Geometry check sheet. Reference: the model listing, model coordinates, mm. Give positions to 0.01 mm unless a question says otherwise; leave off trailing zeros. Write each loop counter-clockwise with the first axis right and the second up, starting at its lowest first coordinate (ties: lowest second). Pieces come first, ordered by that corner, then holes. Notation, with made-up numbers: (4, 46) -> (57, 46) arc R13 cw to (57, 55) -> close; hole circle Ø4 at (58, 70). An arc over 180 degrees is marked (long way). One line per item, written item: value.
from build123d import *

# Parameters (mm, degrees)
ESQUISSE1_W             = 10
ESQUISSE1_H             = 10
BOSS_EXTRU_1_DEPTH      = 95
ESQUISSE2_W             = 10
ESQUISSE2_H             = 5
BOSS_EXTRU_2_DEPTH      = 0.01
ESQUISSE3_W             = 10
ESQUISSE3_H             = 5
BOSS_EXTRU_3_DEPTH      = 0.01
ENL_V_MAT_EXTRU_2_DEPTH = 96.656155578


with BuildPart() as part:
    # Esquisse1 → Boss.-Extru.1 (new body)
    with BuildSketch(Plane.XY):
        Rectangle(ESQUISSE1_W, ESQUISSE1_H)
    extrude(amount=BOSS_EXTRU_1_DEPTH)

    # Esquisse2 → Boss.-Extru.2 (add)
    with BuildSketch(Plane(origin=(0, 5, 0), x_dir=(1, 0, 0), z_dir=(0, 1, 0))):
        with Locations((0, -92.5)):
            Rectangle(ESQUISSE2_W, ESQUISSE2_H)
    extrude(amount=BOSS_EXTRU_2_DEPTH)

    # Esquisse3 → Boss.-Extru.3 (add)
    with BuildSketch(Plane.XZ.offset(5)):
        with Locations((0, 2.5)):
            Rectangle(ESQUISSE3_W, ESQUISSE3_H)
    extrude(amount=BOSS_EXTRU_3_DEPTH)

    # Esquisse6 → Enlèv. mat.-Extru.2 (cut, through all)
    with BuildSketch(Plane(origin=(5, 0, 0), x_dir=(0, 0, -1), z_dir=(1, 0, 0))):
        with BuildLine():
            ThreePointArc((-27.625, 1.931491673), (-35.125, -0.005), (-27.625, -1.941491673))
            ThreePointArc((-27.625, -1.941491673), (-20.125, -0.005), (-27.625, 1.931491673))
        make_face()
    extrude(amount=-ENL_V_MAT_EXTRU_2_DEPTH, mode=Mode.SUBTRACT)


solid = part.part
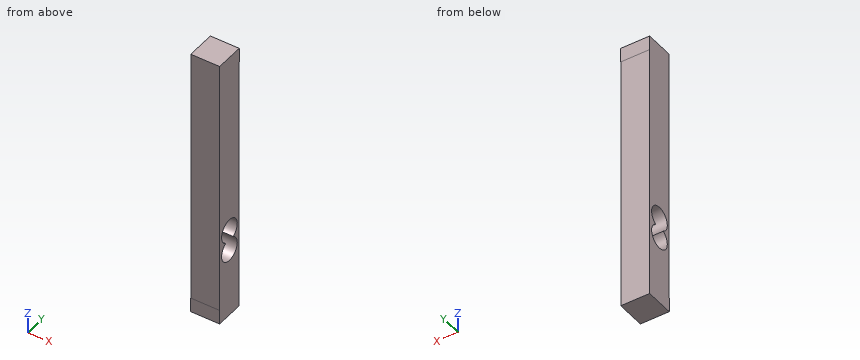
1) Depth check by flat-ended pin: pin 1 Ø5 at (x, z) = (-0.5, 62) entering from +Y; pin 2 Ø2 at (x, z) = (1.5, 72) entering from -Y. Enter the tip coordinate at first touch or a pass-through.
Verdict:
pin 1: y = 5
pin 2: y = -5
2) Scan lines: probe 1 along Z at (x, y) = (-4, 2.5); probe 2 along Z at (x, y) = (3.5, -3.5); probe 3 along Y at (x, z) = (2.25, 89.5). Record each from-to range of solid material in increasing order.
Verdict:
probe 1: 0 to 21.01, 27.24 to 28.01, 34.24 to 95
probe 2: 0 to 22.18, 26.07 to 29.18, 33.07 to 95
probe 3: -5 to 5
3) Sectioned sample at A-A on y = 0. Record the cut outline in (x, z) (3 decimals), plus the area to 3 significant figures.
Verdict:
outline: (-5, 0) -> (5, 0) -> (5, 20.125) -> (-5, 20.125) -> close; (-5, 35.125) -> (5, 35.125) -> (5, 95) -> (-5, 95) -> close
area: 800 mm^2
